```python
from build123d import *

# Parameters (mm, degrees)
SKETCH1_R           = 5
SKETCH1_W           = 3
SKETCH1_H           = 3
BOSS_EXTRUDE1_DEPTH = 6.3
SKETCH2_R           = 3.15
SKETCH2_W           = 3
SKETCH2_H           = 3
BOSS_EXTRUDE2_DEPTH = 1.55
SKETCH3_R           = 3.15
SKETCH3_W           = 3
SKETCH3_H           = 3
BOSS_EXTRUDE3_DEPTH = 1.55


with BuildPart() as part:
    # Sketch1 → Boss-Extrude1 (new body)
    with BuildSketch(Plane.XY):
        Circle(SKETCH1_R)
        Rectangle(SKETCH1_W, SKETCH1_H, mode=Mode.SUBTRACT)
        with BuildLine():
            ThreePointArc((-4.942448008, -0.756444105), (-5, 0), (-4.942448008, 0.756444105))
            Line((-4.942448008, 0.756444105), (-5, 0.75))
            Line((-5, 0.75), (-7.232738071, 0.5))
            Line((-7.232738071, 0.5), (-7.232738071, -0.5))
            Line((-7.232738071, -0.5), (-5, -0.75))
            Line((-5, -0.75), (-4.942448008, -0.756444105))
        make_face()
        with BuildLine():
            ThreePointArc((-4.658507585, 1.816124193), (-4.330127019, 2.5), (-3.90206348, 3.126323815))
            Line((-3.90206348, 3.126323815), (-3.955127019, 3.149519053))
            Line((-3.955127019, 3.149519053), (-6.013734908, 4.049381737))
            Line((-6.013734908, 4.049381737), (-6.513734908, 3.183356333))
            Line((-6.513734908, 3.183356333), (-4.705127019, 1.850480947))
            Line((-4.705127019, 1.850480947), (-4.658507585, 1.816124193))
        make_face()
        with BuildLine():
            ThreePointArc((-3.126323815, 3.90206348), (-2.5, 4.330127019), (-1.816124193, 4.658507585))
            Line((-1.816124193, 4.658507585), (-1.850480947, 4.705127019))
            Line((-1.850480947, 4.705127019), (-3.183356333, 6.513734908))
            Line((-3.183356333, 6.513734908), (-4.049381737, 6.013734908))
            Line((-4.049381737, 6.013734908), (-3.149519053, 3.955127019))
            Line((-3.149519053, 3.955127019), (-3.126323815, 3.90206348))
        make_face()
        with BuildLine():
            Line((0.5, 7.232738071), (-0.5, 7.232738071))
            Line((-0.5, 7.232738071), (-0.75, 5))
            Line((-0.75, 5), (-0.756444105, 4.942448008))
            ThreePointArc((-0.756444105, 4.942448008), (0, 5), (0.756444105, 4.942448008))
            Line((0.756444105, 4.942448008), (0.75, 5))
            Line((0.75, 5), (0.5, 7.232738071))
        make_face()
        with BuildLine():
            Line((1.850480947, 4.705127019), (1.816124193, 4.658507585))
            ThreePointArc((1.816124193, 4.658507585), (2.5, 4.330127019), (3.126323815, 3.90206348))
            Line((3.126323815, 3.90206348), (3.149519053, 3.955127019))
            Line((3.149519053, 3.955127019), (4.049381737, 6.013734908))
            Line((4.049381737, 6.013734908), (3.183356333, 6.513734908))
            Line((3.183356333, 6.513734908), (1.850480947, 4.705127019))
        make_face()
        with BuildLine():
            Line((3.955127019, 3.149519053), (3.90206348, 3.126323815))
            ThreePointArc((3.90206348, 3.126323815), (4.330127019, 2.5), (4.658507585, 1.816124193))
            Line((4.658507585, 1.816124193), (4.705127019, 1.850480947))
            Line((4.705127019, 1.850480947), (6.513734908, 3.183356333))
            Line((6.513734908, 3.183356333), (6.013734908, 4.049381737))
            Line((6.013734908, 4.049381737), (3.955127019, 3.149519053))
        make_face()
        with BuildLine():
            Line((5, 0.75), (4.942448008, 0.756444105))
            ThreePointArc((4.942448008, 0.756444105), (4.985591241, 0.379315144), (5, 0))
            ThreePointArc((5, 0), (4.985591241, -0.379315144), (4.942448008, -0.756444105))
            Line((4.942448008, -0.756444105), (5, -0.75))
            Line((5, -0.75), (7.232738071, -0.5))
            Line((7.232738071, -0.5), (7.232738071, 0.5))
            Line((7.232738071, 0.5), (5, 0.75))
        make_face()
        with BuildLine():
            Line((4.705127019, -1.850480947), (4.658507585, -1.816124193))
            ThreePointArc((4.658507585, -1.816124193), (4.330127019, -2.5), (3.90206348, -3.126323815))
            Line((3.90206348, -3.126323815), (3.955127019, -3.149519053))
            Line((3.955127019, -3.149519053), (6.013734908, -4.049381737))
            Line((6.013734908, -4.049381737), (6.513734908, -3.183356333))
            Line((6.513734908, -3.183356333), (4.705127019, -1.850480947))
        make_face()
        with BuildLine():
            Line((3.149519053, -3.955127019), (3.126323815, -3.90206348))
            ThreePointArc((3.126323815, -3.90206348), (2.5, -4.330127019), (1.816124193, -4.658507585))
            Line((1.816124193, -4.658507585), (1.850480947, -4.705127019))
            Line((1.850480947, -4.705127019), (3.183356333, -6.513734908))
            Line((3.183356333, -6.513734908), (4.049381737, -6.013734908))
            Line((4.049381737, -6.013734908), (3.149519053, -3.955127019))
        make_face()
        with BuildLine():
            ThreePointArc((0.756444105, -4.942448008), (0, -5), (-0.756444105, -4.942448008))
            Line((-0.756444105, -4.942448008), (-0.75, -5))
            Line((-0.75, -5), (-0.5, -7.232738071))
            Line((-0.5, -7.232738071), (0.5, -7.232738071))
            Line((0.5, -7.232738071), (0.75, -5))
            Line((0.75, -5), (0.756444105, -4.942448008))
        make_face()
        with BuildLine():
            ThreePointArc((-1.816124193, -4.658507585), (-2.5, -4.330127019), (-3.126323815, -3.90206348))
            Line((-3.126323815, -3.90206348), (-3.149519053, -3.955127019))
            Line((-3.149519053, -3.955127019), (-4.049381737, -6.013734908))
            Line((-4.049381737, -6.013734908), (-3.183356333, -6.513734908))
            Line((-3.183356333, -6.513734908), (-1.850480947, -4.705127019))
            Line((-1.850480947, -4.705127019), (-1.816124193, -4.658507585))
        make_face()
        with BuildLine():
            ThreePointArc((-3.90206348, -3.126323815), (-4.330127019, -2.5), (-4.658507585, -1.816124193))
            Line((-4.658507585, -1.816124193), (-4.705127019, -1.850480947))
            Line((-4.705127019, -1.850480947), (-6.513734908, -3.183356333))
            Line((-6.513734908, -3.183356333), (-6.013734908, -4.049381737))
            Line((-6.013734908, -4.049381737), (-3.955127019, -3.149519053))
            Line((-3.955127019, -3.149519053), (-3.90206348, -3.126323815))
        make_face()
    extrude(amount=BOSS_EXTRUDE1_DEPTH)

    # Sketch2 → Boss-Extrude2 (add)
    with BuildSketch(Plane.XY.offset(6.3)):
        Circle(SKETCH2_R)
        Rectangle(SKETCH2_W, SKETCH2_H, mode=Mode.SUBTRACT)
    extrude(amount=BOSS_EXTRUDE2_DEPTH)

    # Sketch3 → Boss-Extrude3 (add)
    with BuildSketch(Plane(origin=(0, 0, 0), x_dir=(-1, 0, 0), z_dir=(0, 0, -1))):
        Circle(SKETCH3_R)
        Rectangle(SKETCH3_W, SKETCH3_H, mode=Mode.SUBTRACT)
    extrude(amount=BOSS_EXTRUDE3_DEPTH)


solid = part.part
```
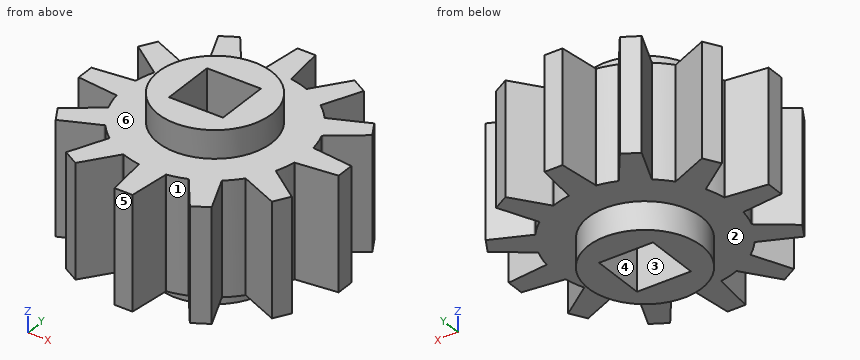
Model file for the job. Use its own axes, mm. Face numbers are marked on the shaded views. A direction names the side the tool comes from. Round coordinates to 2 decimals unless told otherwise and drop trailing zeros. Loops run counter-clockwise (first coordinate to the right, second up) from the corner with the lowest first, then second, coordinate; pieces in that order, holes last. Notation, with made-up numbers: M 1,87.5 L 7,87.5 A8 ccw 7,97.5 Z; hole C 62.5,18.5 d5. An arc over 180 degrees is marked long. Put each result on its own line as item: value. Start each with the question number.
Item 1: 3-axis set-ups, long thin cutter, end or side, ignore diameter. For the marked faces 1, 2 and 3: which of +Z, -Z, +X, -X, +Y, -Y reach the whole face in a straight line?
Item 2: Drill centre lines: line 1 along X through (y, z) = (3.25, 3.25) (3 decimals); line 2 along X through (y, z) = (5.5, 3); line 3 along X through (y, z) = (0, 5.75). Where is each one in solid material? Low to high.
Item 3: Mould opens along Y. For the marked faces 4, 5 and 6 say: released by +Y, released by -Y, zero draft, split by the parting line, or undercut.
Item 4: Cut at C-C (z = 7). List the corners of the cut face in (x, y).
Item 5: Cut at D-D (x = -5.5). List the corners of the cut face in (y, z), then the cut area to 3 significant figures.
Item 6: Cut at A-A (x = 0). List the corners of the cut face in (y, z), then the cut area to 3 significant figures.
Item 7: Drop a flat-ended pin along its axis: P1, Ø4, axis at x = 4.5, z = 1.5, coming from the +Y side. Give the stop position or say it passes through.
Answer block:
1. face 1: +Z, -Z, -Y
1. face 2: -Z
1. face 3: +Z, -Z
2. line 1: -6.475 to -4.185, -3.8 to 3.8, 4.185 to 6.475
2. line 2: -3.82 to -2.44, -0.69 to 0.69, 2.44 to 3.82
2. line 3: -7.23 to -1.5, 1.5 to 7.23
3. face 4: undercut
3. face 5: released by -Y
3. face 6: zero draft
4. outline: C 0,0 d6.3; hole M -1.5,-1.5 L 1.5,-1.5 L 1.5,1.5 L -1.5,1.5 Z
5. outline: M -3.82,0 L -2.44,0 L -2.44,6.3 L -3.82,6.3 Z; M -0.69,0 L 0.69,0 L 0.69,6.3 L -0.69,6.3 Z; M 2.44,0 L 3.82,0 L 3.82,6.3 L 2.44,6.3 Z
5. area: 26.2 mm2
6. outline: M -7.23,0 L -3.15,0 L -3.15,-1.55 L -1.5,-1.55 L -1.5,7.85 L -3.15,7.85 L -3.15,6.3 L -7.23,6.3 Z; M 1.5,-1.55 L 3.15,-1.55 L 3.15,0 L 7.23,0 L 7.23,6.3 L 3.15,6.3 L 3.15,7.85 L 1.5,7.85 Z
6. area: 82.5 mm2
7. P1: y = 6.51
